Work out the finished part from the listing and answer in its coordinate system (mm). Face numbers are marked on the shaded views. Give positions to 0.01 mm unless a question says otherwise; leave off trailing zeros. Loops run counter-clockwise (first coordinate to the right, second up) from the corner with the lowest first, then second, coordinate; pieces in that order, holes last. Notation, with made-up numbers: (-35, -6.75) - (-17, -6.75) arc R9 ccw to (-17, 1.25) - close; hole circle Ø11 at (-8.5, 4). An arc over 180 degrees is marked (long way). One line per question, with ' | ' between items. Start each with the question number.
1. Section C-C (y = 101) is taken. Determine the outline of the cut face in (x, z), plus the area to 3 significant figures.
2. Section B-B (x = -28) is taken. Determine the outline of the cut face in (y, z), plus the area to 3 significant figures.
3. Section A-A (z = 7.25) is taken. Determine the outline of the cut face in (x, y).
4. Find the intervals of material crossed by line 1 (Y direction, x = -112, z = 6); line 2 (X direction, y = 37, z = 4.75); line 3 (Z direction, x = -55.5, y = 54.5), in increasing order.
5. Each of these flat-tipped pins is pushed along its axis until it touches: pin 1 (8 mm diameter, centred on y = 67, z = 12, fed in from +X); pin 2 (1 mm diameter, centred on x = -53.5, y = 39, fed in from -Z). Where does it stop, or does it pass through?
6. For a pull along X with two mould halves and no side action, classify the marked faces 1, 2 and 3 as released by +X, released by -X, zero draft, split by the parting line, or undercut.
from build123d import *

# Parameters (mm, degrees)
SKETCH1_W           = 160
SKETCH1_H           = 130
BOSS_EXTRUDE1_DEPTH = 20
CUT_EXTRUDE1_DEPTH  = 10


with BuildPart() as part:
    # Sketch1 → Boss-Extrude1 (new body)
    with BuildSketch(Plane.XY):
        with Locations((-80, 65)):
            Rectangle(SKETCH1_W, SKETCH1_H)
    extrude(amount=BOSS_EXTRUDE1_DEPTH)

    # Sketch2 → Cut-Extrude1 (cut)
    with BuildSketch(Plane(origin=(0, 0, 0), x_dir=(-1, 0, 0), z_dir=(0, 0, -1))):
        with BuildLine():
            Line((150, 110), (150, 20))
            ThreePointArc((150, 20), (147.071067812, 12.928932188), (140, 10))
            Line((140, 10), (20, 10))
            ThreePointArc((20, 10), (12.928932188, 12.928932188), (10, 20))
            Line((10, 20), (10, 110))
            ThreePointArc((10, 110), (12.928932188, 117.071067812), (20, 120))
            Line((20, 120), (140, 120))
            ThreePointArc((140, 120), (147.071067812, 117.071067812), (150, 110))
        make_face()
    extrude(amount=-CUT_EXTRUDE1_DEPTH, mode=Mode.SUBTRACT)


solid = part.part
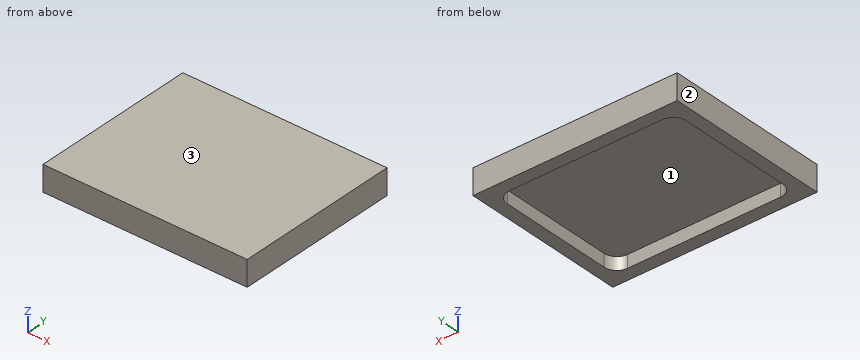
Conclusion:
1) outline: (-160, 0) - (-150, 0) - (-150, 10) - (-10, 10) - (-10, 0) - (0, 0) - (0, 20) - (-160, 20) - close | area: 1,800 mm²
2) outline: (0, 0) - (10, 0) - (10, 10) - (120, 10) - (120, 0) - (130, 0) - (130, 20) - (0, 20) - close | area: 1,500 mm²
3) outline: (-160, 0) - (0, 0) - (0, 130) - (-160, 130) - close; hole (-150, 20) arc R10 ccw to (-140, 10) - (-20, 10) arc R10 ccw to (-10, 20) - (-10, 110) arc R10 ccw to (-20, 120) - (-140, 120) arc R10 ccw to (-150, 110) - close
4) line 1: 0 to 10, 120 to 130 | line 2: -160 to -150, -10 to 0 | line 3: 10 to 20
5) pin 1: x = 0 | pin 2: z = 10
6) face 1: undercut | face 2: released by -X | face 3: zero draft
